For this review, use the dimensioned drawing (mm, ordinates from the lowest corner) and the shaded views. Give positions to 0.01 mm unless a question says otherwise; leave off trailing zeros. Write each loop counter-clockwise with the first axis right and the second up, starting at its lowest first coordinate (ties: lowest second). Pieces come first, ordered by that corner, then holes. Notation, with made-up numbers: M 80.25,89.5 L 123.25,89.5 A22 ccw 123.25,102.5 Z; hole C 41.5,-4 d6. An arc over 180 degrees is marked long. Answer in a Markdown table with one row per item.
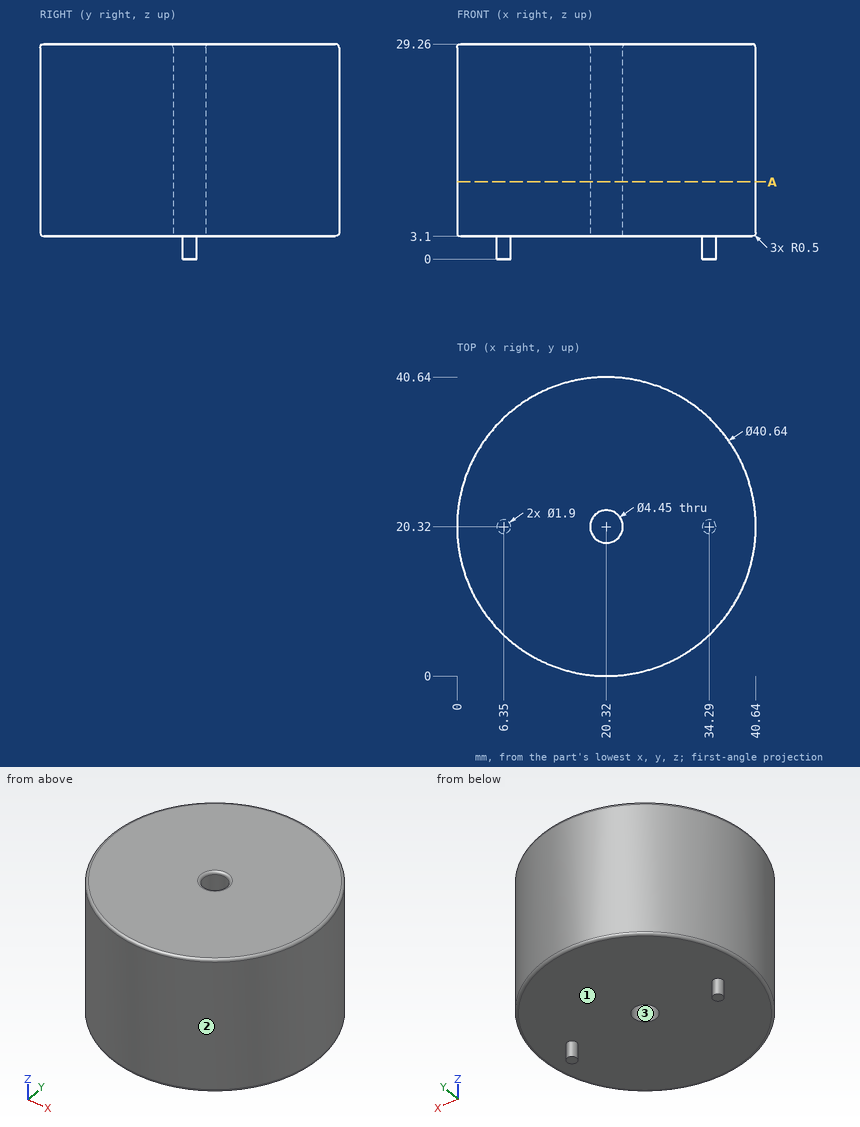
1) To check wall thickness, follow probe 1 along Y at (x, z) = (20.32, 14.5) (3 decimals); probe 2 along Z at (x, y) = (33, 33); probe 3 along X at (y, z) = (29, 3.25). State the ranges of each line that lie inside material, in increasing order. Write a range as [from, to].
Geometry says:
| item | result |
|---|---|
| probe 1 | [0, 18.095], [22.545, 40.64] |
| probe 2 | [3.1, 29.26] |
| probe 3 | [2.11, 38.53] |
2) The part is to be moulded in two halves that separate along Y. For the marked faces 1, 2 and 3, say which applies: released by +Y, released by -Y, zero draft, split by the parting line, or undercut.
Geometry says:
| item | result |
|---|---|
| face 1 | zero draft |
| face 2 | split by the parting line |
| face 3 | undercut |
3) Insertion check: P1, Ø12, axis at x = 21.5, z = 5, coming from the -Y side; P2, Ø1.5, axis at x = 9.5, z = 6.5, coming from the -Y side; P3, Ø10, axis at x = 8, z = 6.5, coming from the -Y side. Each pin has a flat end and moves straight along its axis. Give the tip position at first contact, or say it passes through.
Geometry says:
| item | result |
|---|---|
| P1 | y = 0 |
| P2 | y = 2.67 |
| P3 | y = 1.36 |
4) Add section A-A (z = 10.5). Write out the cut boundary in (x, y) (3 decimals).
Geometry says:
| item | result |
|---|---|
| outline | C 20.32,20.32 d40.64; hole C 20.32,20.32 d4.45 |
